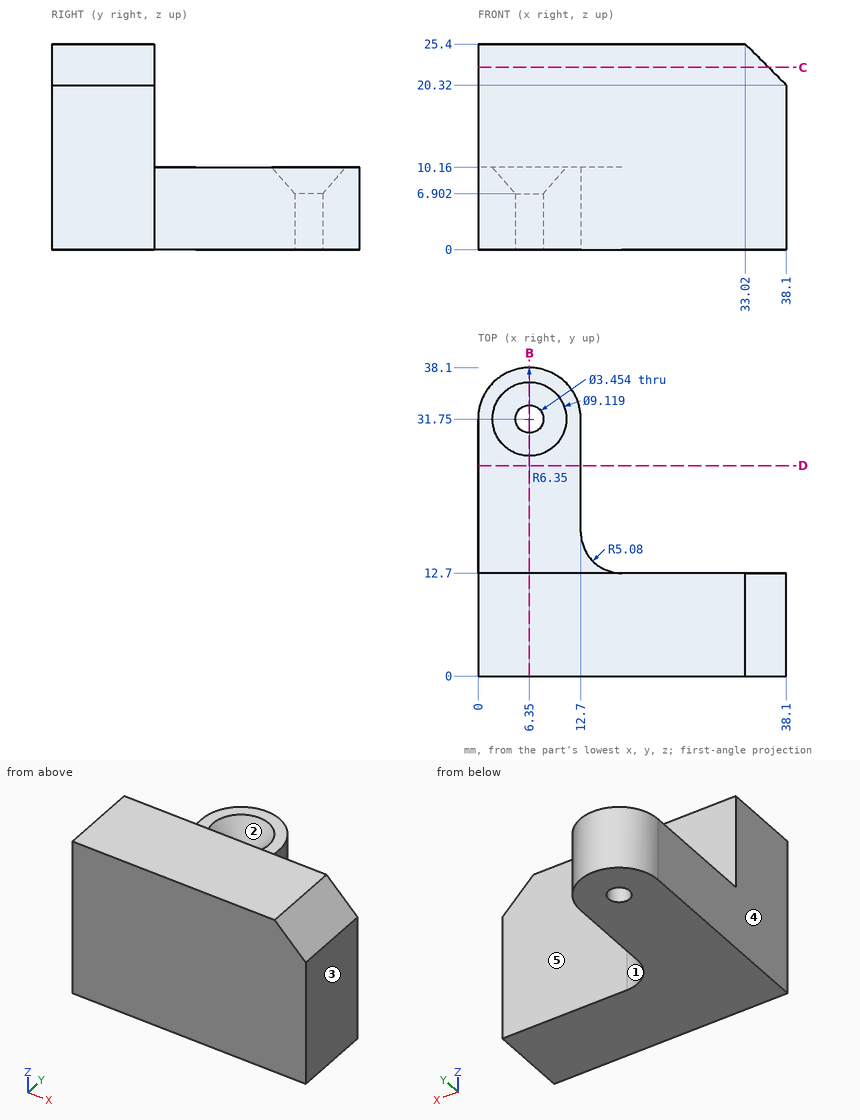
Source: three-view drawing plus pictorial views. Frame: mm from the lowest corner of the part. A direction names the side the tool comes from. Round coordinates to 2 decimals unless told otherwise and drop trailing zeros. Order: outer loops, then holes, each group sorted by start corner. A loop starts at its lowest first (then second) coordinate and runs counter-clockwise, first axis right, second up. Notation, with made-up numbers: (25, 80.25) - (66, 80.25) arc R12 ccw to (66, 96.25) - close; hole circle Ø4 at (68, 73.25). An arc over 180 degrees is marked (long way). Use a Markdown table: item, result.
1. Section C-C on z = 22.5. Return the cut outline in (x, y).
Evaluation:
| item | result |
|---|---|
| outline | (0, 0) - (35.92, 0) - (35.92, 12.7) - (0, 12.7) - close |
2. Mould query, pull axis Y, two halves, no side actions, for the marked faces 1, 2 and 3. Classes: +Y half, -Y half, draft (parallel to the pull), parting line (faces both ways), or undercut.
Evaluation:
| item | result |
|---|---|
| face 1 | +Y half |
| face 2 | undercut |
| face 3 | draft |
3. Material intervals for probe 1 along X at (y, z) = (31.75, 3.75); probe 2 along Y at (x, z) = (6.35, 2); probe 3 along Y at (x, z) = (4, 11.5), sorted ascending.
Evaluation:
| item | result |
|---|---|
| probe 1 | 0 to 4.62, 8.08 to 12.7 |
| probe 2 | 0 to 30.02, 33.48 to 38.1 |
| probe 3 | 0 to 12.7 |
4. Section B-B on x = 6.35. Return the cut outline in (y, z).
Evaluation:
| item | result |
|---|---|
| outline | (0, 0) - (30.02, 0) - (30.02, 6.9) - (27.19, 10.16) - (12.7, 10.16) - (12.7, 25.4) - (0, 25.4) - close; (33.48, 0) - (38.1, 0) - (38.1, 10.16) - (36.31, 10.16) - (33.48, 6.9) - close |
5. Access query for the marked faces 4 and 5. Directions: +Z, -Z, +X, -X, +Y, -Y. A direction counts if a zero-diameter tool reaches every point of the face in a straight line with its end or side. Return the directions, or none.
Evaluation:
| item | result |
|---|---|
| face 4 | +Z, -Z, -X, +Y, -Y |
| face 5 | +Z, +X, +Y |
6. First-contact query: pin 1 (2 mm diameter, centred on x = 14, z = 11.5, fed in from +Y); pin 2 (5.5 mm diameter, centred on x = 10.5, y = 21, fed in from +Z); pin 3 (3 mm diameter, centred on y = 24, z = 5.5, fed in from +X); pin 4 (1.5 mm diameter, centred on y = 22, z = 11, fed in from +X). Flat tips, straight axial feed; report the tip coordinate or a pass-through.
Evaluation:
| item | result |
|---|---|
| pin 1 | y = 12.7 |
| pin 2 | z = 10.16 |
| pin 3 | x = 12.7 |
| pin 4 | through |
7. Section D-D on y = 26. Return the cut outline in (x, z), then the cut area to 3 significant figures.
Evaluation:
| item | result |
|---|---|
| outline | (0, 0) - (12.7, 0) - (12.7, 10.16) - (0, 10.16) - close |
| area | 129 mm^2 |
